Work out the finished part from the listing and answer in its coordinate system (mm). A direction names the side the tool comes from. Give positions to 0.01 mm unless a question says otherwise; leave off trailing zeros. Order: outer loops, then holes, each group sorted by start corner. A loop starts at its lowest first (then second) coordinate and runs counter-clockwise, first axis right, second up. Notation, with made-up numbers: (56, 17) -> (101, 17) arc R35 ccw to (101, 53) -> close; hole circle Ø10 at (-33.5, 19.25). An arc over 180 degrees is marked (long way). Answer as CSV lines item,"result". Start each with the question number.
1. A cutting plane is placed at A-A (z = 10). Give the vertices of the cut face in (x, y).
2. A cutting plane is placed at D-D (y = -71.4). Give the vertices of the cut face in (x, z), then the cut area to 3 significant figures.
3. For faces 1 (the flat face through (0, -1, 2.2)), 2 (the flat face through (18.75, -1, 10)), 3 (the cylindrical face through (17.67, -65.44, 11.88)), determine the directions among +Z, -Z, +X, -X, +Y, -Y from which every point of the face is accessible in a straight line to the end or side of a thin tool.
4. A flat-ended cylindrical pin translates along its axis: pin 1 (4.5 mm diameter, centred on x = -6, z = 12, fed in from -Y). Find the tip coordinate at first contact, or state that the pin passes through.
5. A cutting plane is placed at B-B (y = -48). Give the vertices of the cut face in (x, z).
6. A cutting plane is placed at C-C (x = -8.5). Give the vertices of the cut face in (y, z), then the cut area to 3 significant figures.
7. Find the intervals of material crossed by L1, parallel to X at y = 69, z = 7.25; L2, parallel to Z at x = 17, y = -71; L3, parallel to Z at x = 6, y = 69.5, in increasing order.
8. For a pull along Z with two mould halves and no side action, classify faces 4 (the flat face through (-18.75, -1, 10)), 5 (the flat face through (0, 85.85, 10)), 6 (the flat face through (0, 1, 0)), 7 (the flat face through (-16.55, -1, 10)) as released by +Z, released by -Z, zero draft, split by the parting line, or undercut.
from build123d import *

# Parameters (mm, degrees)
SKETCH_W        = 37.5
SKETCH_H        = 172.3
PAD_DEPTH       = 20
SKETCH001_W     = 33.1
SKETCH001_H     = 15.6
POCKET_DEPTH    = 172
SKETCH002_R     = 6.25
POCKET001_DEPTH = 10


with BuildPart() as part:
    # Sketch → Pad (new body)
    with BuildSketch(Plane.XY):
        Rectangle(SKETCH_W, SKETCH_H)
    extrude(amount=PAD_DEPTH)

    # Sketch001 (on Face1 of Pad) → Pocket (cut)
    with BuildSketch(Plane.XZ.offset(86.15)):
        with Locations((0, 10)):
            Rectangle(SKETCH001_W, SKETCH001_H)
    extrude(amount=-POCKET_DEPTH, mode=Mode.SUBTRACT)

    # Sketch002 (on Face5 of Pocket) → Pocket001 (cut)
    with BuildSketch(Plane.YZ.offset(18.75)):
        with Locations((-71.4, 10)):
            Circle(SKETCH002_R)
    extrude(amount=-POCKET001_DEPTH, mode=Mode.SUBTRACT)


solid = part.part
Answer sheet:
1,outline,"(-18.75, -86.15) -> (-16.55, -86.15) -> (-16.55, 85.85) -> (16.55, 85.85) -> (16.55, -65.15) -> (18.75, -65.15) -> (18.75, 86.15) -> (-18.75, 86.15) -> close; (16.55, -86.15) -> (18.75, -86.15) -> (18.75, -77.65) -> (16.55, -77.65) -> close"
2,outline,"(-18.75, 0) -> (18.75, 0) -> (18.75, 3.75) -> (16.55, 3.75) -> (16.55, 2.2) -> (-16.55, 2.2) -> (-16.55, 17.8) -> (16.55, 17.8) -> (16.55, 16.25) -> (18.75, 16.25) -> (18.75, 20) -> (-18.75, 20) -> close"
2,area,"206 mm^2"
3,face 1,"-Y"
3,face 2,"+Z, -Z, +X, +Y, -Y"
3,face 3,"+X"
4,pin 1,"stops at y = 85.85"
5,outline,"(-18.75, 0) -> (18.75, 0) -> (18.75, 20) -> (-18.75, 20) -> close; hole (-16.55, 2.2) -> (16.55, 2.2) -> (16.55, 17.8) -> (-16.55, 17.8) -> close"
6,outline,"(-86.15, 0) -> (86.15, 0) -> (86.15, 20) -> (-86.15, 20) -> (-86.15, 17.8) -> (85.85, 17.8) -> (85.85, 2.2) -> (-86.15, 2.2) -> close"
6,area,"763 mm^2"
7,L1,"x = -18.75 to -16.55, 16.55 to 18.75"
7,L2,"z = 0 to 3.76, 16.24 to 20"
7,L3,"z = 0 to 2.2, 17.8 to 20"
8,face 4,"zero draft"
8,face 5,"undercut"
8,face 6,"released by -Z"
8,face 7,"undercut"
